Here's how the part is built. I have some questions about the finished solid (model axes, mm). A direction names the side the tool comes from. Round coordinates to 2 decimals unless told otherwise and drop trailing zeros. Order: outer loops, then holes, each group sorted by start corner. A loop starts at its lowest first (then second) coordinate and runs counter-clockwise, first axis right, second up. Notation, with made-up numbers: (-3.75, 47.25) -> (14.25, 47.25) arc R23 ccw to (14.25, 83.25) -> close; hole circle Ø8 at (6.25, 45.25). An arc over 180 degrees is marked (long way). Use a Markdown table: item, result. Add a question column.
(1) I want a section at A-A, the plane z = 17. Please give me the cut outline in (x, y), then the cut area to 3 significant figures.
(2) On a 3-axis mill with a long thin cutter (end or side, diameter ignored), from which of +Z, -Z, +X, -X, +Y, -Y can I reach the whole of each face in a straight line? I mean faces 1 (the face through (2, 5, 0)), 2 (the face through (12, 0, 5)), 3 (the face through (-7, -2.5, 15)). Say none if no direction works.
(3) I want a section at B-B, the plane x = -2.75. Please give me the cut outline in (y, z).
(4) Thinking about a two-plate mould opening in X: for faces 4 (the face through (17, -8, 12)), 5 (the face through (-4, -3, 10)), 6 (the face through (8, 10, 12)), which applies, pulls with the +X half, pulls with the -X half, needs draft (parallel to the pull), parting line crosses it, or undercut?
(5) I want a section at D-D, the plane y = 3.5. Please give me the cut outline in (x, z).
(6) If I drill on probe 1 along Y at (x, z) = (0, 15.75); probe 2 along X at (y, z) = (0, 6.5), over which ranges is the centre line in solid material (lowest first)?
(7) I want a section at C-C, the plane x = 14.5. Please give me the cut outline in (y, z), then the cut area to 3 significant figures.
(8) I'm going to push flat-ended pins straight in: P1, Ø12, axis at y = 3.5, z = 2.5, coming from the +X side; P2, Ø4, axis at x = 14, y = 0, coming from the +Z side; P3, Ø5, axis at x = -6.5, z = 16, coming from the +Y side; P4, Ø1.6, axis at x = -8, z = 13.5, coming from the -Y side. Where does each tip first touch, or does it pass through?
from build123d import *
from build123d import SkipClean  # not in build123d's __all__

# Parameters (mm, degrees)
F0_R     = 5
F1_DEPTH = 20
F2_DEPTH = 20
F3_W     = 5
F3_H     = 10
F4_DEPTH = 30
F5_DEPTH = 5


with BuildPart() as f1:
    # F0 (on Top) → F1 (new body)
    with BuildSketch(Plane.XY):
        with BuildLine():
            ThreePointArc((0, -10), (7.0710678119, -7.0710678119), (10, 0))
            ThreePointArc((10, 0), (7.0710678119, 7.0710678119), (0, 10))
            ThreePointArc((0, 10), (-10, 0), (0, -10))
        make_face()
        Circle(F0_R, mode=Mode.SUBTRACT)
    extrude(amount=F1_DEPTH)

    # F0 (on Top) → F2 (join)
    with BuildSketch(Plane.XY):
        with BuildLine():
            ThreePointArc((0, 10), (7.0710678119, 7.0710678119), (10, 0))
            ThreePointArc((10, 0), (7.0710678119, -7.0710678119), (0, -10))
            Line((0, -10), (15, -10))
            Line((15, -10), (20, -5))
            Line((20, -5), (20, 5))
            Line((20, 5), (15, 10))
            Line((15, 10), (0, 10))
        make_face()
    extrude(amount=F2_DEPTH)

    # F3 (on face) → F4 (cut)
    with BuildSketch(Plane.YZ.offset(20)):
        with Locations((0, 15)):
            Rectangle(F3_W, F3_H)
    extrude(amount=-F4_DEPTH, mode=Mode.SUBTRACT)

    # F0 (on Top) → F5 (cut)
    with BuildSketch(Plane.XY):
        with BuildLine():
            ThreePointArc((0, 10), (7.0710678119, 7.0710678119), (10, 0))
            ThreePointArc((10, 0), (7.0710678119, -7.0710678119), (0, -10))
            Line((0, -10), (15, -10))
            Line((15, -10), (20, -5))
            Line((20, -5), (20, 5))
            Line((20, 5), (15, 10))
            Line((15, 10), (0, 10))
        make_face()
    with SkipClean():  # cleaning this boolean's faces spoils the solid; the shape is the same uncleaned
        extrude(amount=F5_DEPTH, mode=Mode.SUBTRACT)


solid = f1.part
Taken from the geometry:
| question | item | result |
|---|---|---|
| 1 | outline | (-9.68, -2.5) arc R10 ccw to (0, -10) -> (15, -10) -> (20, -5) -> (20, -2.5) -> (4.33, -2.5) arc R5 cw to (-4.33, -2.5) -> close; (-9.68, 2.5) -> (-4.33, 2.5) arc R5 cw to (4.33, 2.5) -> (20, 2.5) -> (20, 5) -> (15, 10) -> (0, 10) arc R10 ccw to start |
| 1 | area | 352 mm2 |
| 2 | face 1 | -Z, +X, -X, +Y, -Y |
| 2 | face 2 | -Z, +X |
| 2 | face 3 | +Z, +X, -X |
| 3 | outline | (-9.61, 0) -> (-4.18, 0) -> (-4.18, 20) -> (-9.61, 20) -> close; (4.18, 0) -> (9.61, 0) -> (9.61, 20) -> (4.18, 20) -> close |
| 4 | face 4 | pulls with the +X half |
| 4 | face 5 | undercut |
| 4 | face 6 | needs draft |
| 5 | outline | (-9.37, 0) -> (-3.57, 0) -> (-3.57, 20) -> (-9.37, 20) -> close; (3.57, 0) -> (9.37, 0) -> (9.37, 5) -> (20, 5) -> (20, 20) -> (3.57, 20) -> close |
| 6 | probe 1 | y = -10 to -5, 5 to 10 |
| 6 | probe 2 | x = -10 to -5, 5 to 20 |
| 7 | outline | (-10, 5) -> (10, 5) -> (10, 20) -> (2.5, 20) -> (2.5, 10) -> (-2.5, 10) -> (-2.5, 20) -> (-10, 20) -> close |
| 7 | area | 250 mm2 |
| 8 | P1 | stops at x = 20 |
| 8 | P2 | stops at z = 10 |
| 8 | P3 | stops at y = 9.17 |
| 8 | P4 | stops at y = -6.94 |
